Verification items for the finished model (mm, model axes). A direction names the side the tool comes from. Give positions to 0.01 mm unless a question says otherwise; leave off trailing zeros. Write each loop counter-clockwise with the first axis right and the second up, starting at its lowest first coordinate (ties: lowest second). Pieces come first, ordered by that corner, then holes.
from build123d import *

# Parameters (mm, degrees)
F0_R      = 1.2
F1_DEPTH  = 1.5
F2_DEPTH  = 5
F3_DEPTH  = 5.5
F5_DEPTH  = 2
F7_DEPTH  = 2
F8_W      = 10
F8_H      = 5
F9_DEPTH  = 1
F10_R     = 1
F11_DEPTH = 5


# Not quite as in the source:
# - a feature names something its author has since deleted; it is built from what else it names


with BuildPart() as f1:
    # F0 (on Top) → F1 (new body)
    with BuildSketch(Plane.XY):
        with BuildLine():
            Line((14.9310000289, -10.5), (14.9310000289, 10.5))
            ThreePointArc((14.9310000289, 10.5), (13.4665339264, 14.0355339264), (9.931, 15.5000000289))
            Line((9.931, 15.5000000289), (-9.931, 15.5000000289))
            ThreePointArc((-9.931, 15.5000000289), (-13.4665339264, 14.0355339264), (-14.9310000289, 10.5))
            Line((-14.9310000289, 10.5), (-14.9310000289, -10.5))
            ThreePointArc((-14.9310000289, -10.5), (-13.4665339264, -14.0355339264), (-9.931, -15.5000000289))
            Line((-9.931, -15.5000000289), (9.931, -15.5000000289))
            ThreePointArc((9.931, -15.5000000289), (13.4665339264, -14.0355339264), (14.9310000289, -10.5))
        make_face()
        with BuildLine():
            Line((-9.931, 13.5000000289), (-7.581, 13.5000000289))
            Line((-7.581, 13.5000000289), (0.069, 13.5000000289))
            Line((0.069, 13.5000000289), (4.769, 13.5000000289))
            Line((4.769, 13.5000000289), (9.931, 13.5000000289))
            ThreePointArc((9.931, 13.5000000289), (12.052320364, 12.621320364), (12.9310000289, 10.5))
            Line((12.9310000289, 10.5), (12.9310000289, -10.5))
            ThreePointArc((12.9310000289, -10.5), (12.052320364, -12.621320364), (9.931, -13.5000000289))
            Line((9.931, -13.5000000289), (4.769, -13.5000000289))
            Line((4.769, -13.5000000289), (0.069, -13.5000000289))
            Line((0.069, -13.5000000289), (-7.581, -13.5000000289))
            Line((-7.581, -13.5000000289), (-9.931, -13.5000000289))
            ThreePointArc((-9.931, -13.5000000289), (-12.052320364, -12.621320364), (-12.9310000289, -10.5))
            Line((-12.9310000289, -10.5), (-12.9310000289, -8.1))
            Line((-12.9310000289, -8.1), (-12.9310000289, 8.1))
            Line((-12.9310000289, 8.1), (-12.9310000289, 10.5))
            ThreePointArc((-12.9310000289, 10.5), (-12.052320364, 12.621320364), (-9.931, 13.5000000289))
        make_face(mode=Mode.SUBTRACT)
        with BuildLine():
            ThreePointArc((4.769, -10.45), (2.419, -8.1), (0.069, -10.45))
            ThreePointArc((0.069, -10.45), (2.419, -12.8), (4.769, -10.45))
        make_face()
        with Locations((2.419, -10.45)):
            Circle(F0_R, mode=Mode.SUBTRACT)
        with BuildLine():
            ThreePointArc((4.769, 10.45), (2.419, 12.8), (0.069, 10.45))
            ThreePointArc((0.069, 10.45), (2.419, 8.1), (4.769, 10.45))
        make_face()
        with Locations((2.419, 10.45)):
            Circle(F0_R, mode=Mode.SUBTRACT)
        with BuildLine():
            ThreePointArc((-9.931, 8.1), (-11.5927009358, 12.1117009358), (-7.581, 10.45))
            Line((-7.581, 10.45), (-7.581, 13.5000000289))
            Line((-7.581, 13.5000000289), (-9.931, 13.5000000289))
            ThreePointArc((-9.931, 13.5000000289), (-12.052320364, 12.621320364), (-12.9310000289, 10.5))
            Line((-12.9310000289, 10.5), (-12.9310000289, 8.1))
            Line((-12.9310000289, 8.1), (-9.931, 8.1))
        make_face()
        with BuildLine():
            Line((-9.931, -8.1), (-12.9310000289, -8.1))
            Line((-12.9310000289, -8.1), (-12.9310000289, -10.5))
            ThreePointArc((-12.9310000289, -10.5), (-12.052320364, -12.621320364), (-9.931, -13.5000000289))
            Line((-9.931, -13.5000000289), (-7.581, -13.5000000289))
            Line((-7.581, -13.5000000289), (-7.581, -10.45))
            ThreePointArc((-7.581, -10.45), (-11.5927009358, -12.1117009358), (-9.931, -8.1))
        make_face()
        with BuildLine():
            ThreePointArc((-7.581, -10.45), (-8.2692990642, -8.7882990642), (-9.931, -8.1))
            ThreePointArc((-9.931, -8.1), (-11.5927009358, -12.1117009358), (-7.581, -10.45))
        make_face()
        with Locations((-9.931, -10.45)):
            Circle(F0_R, mode=Mode.SUBTRACT)
        with BuildLine():
            Line((0.069, -10.45), (0.069, -13.5000000289))
            Line((0.069, -13.5000000289), (4.769, -13.5000000289))
            Line((4.769, -13.5000000289), (4.769, -10.45))
            ThreePointArc((4.769, -10.45), (2.419, -12.8), (0.069, -10.45))
        make_face()
        with BuildLine():
            ThreePointArc((-9.931, 8.1), (-8.2692990642, 8.7882990642), (-7.581, 10.45))
            ThreePointArc((-7.581, 10.45), (-11.5927009358, 12.1117009358), (-9.931, 8.1))
        make_face()
        with Locations((-9.931, 10.45)):
            Circle(F0_R, mode=Mode.SUBTRACT)
        with BuildLine():
            Line((4.769, 13.5000000289), (0.069, 13.5000000289))
            Line((0.069, 13.5000000289), (0.069, 10.45))
            ThreePointArc((0.069, 10.45), (2.419, 12.8), (4.769, 10.45))
            Line((4.769, 10.45), (4.769, 13.5000000289))
        make_face()
        with BuildLine():
            Line((-7.581, 13.5000000289), (-7.581, 10.45))
            ThreePointArc((-7.581, 10.45), (-8.2692990642, 8.7882990642), (-9.931, 8.1))
            Line((-9.931, 8.1), (-12.9310000289, 8.1))
            Line((-12.9310000289, 8.1), (-12.9310000289, -8.1))
            Line((-12.9310000289, -8.1), (-9.931, -8.1))
            ThreePointArc((-9.931, -8.1), (-8.2692990642, -8.7882990642), (-7.581, -10.45))
            Line((-7.581, -10.45), (-7.581, -13.5000000289))
            Line((-7.581, -13.5000000289), (0.069, -13.5000000289))
            Line((0.069, -13.5000000289), (0.069, -10.45))
            ThreePointArc((0.069, -10.45), (2.419, -8.1), (4.769, -10.45))
            Line((4.769, -10.45), (4.769, -13.5000000289))
            Line((4.769, -13.5000000289), (9.931, -13.5000000289))
            ThreePointArc((9.931, -13.5000000289), (12.052320364, -12.621320364), (12.9310000289, -10.5))
            Line((12.9310000289, -10.5), (12.9310000289, 10.5))
            ThreePointArc((12.9310000289, 10.5), (12.052320364, 12.621320364), (9.931, 13.5000000289))
            Line((9.931, 13.5000000289), (4.769, 13.5000000289))
            Line((4.769, 13.5000000289), (4.769, 10.45))
            ThreePointArc((4.769, 10.45), (2.419, 8.1), (0.069, 10.45))
            Line((0.069, 10.45), (0.069, 13.5000000289))
            Line((0.069, 13.5000000289), (-7.581, 13.5000000289))
        make_face()
    extrude(amount=F1_DEPTH)

    # F0 (on Top) → F2 (join)
    with BuildSketch(Plane.XY):
        with BuildLine():
            ThreePointArc((-9.931, 8.1), (-11.5927009358, 12.1117009358), (-7.581, 10.45))
            Line((-7.581, 10.45), (-7.581, 13.5000000289))
            Line((-7.581, 13.5000000289), (-9.931, 13.5000000289))
            ThreePointArc((-9.931, 13.5000000289), (-12.052320364, 12.621320364), (-12.9310000289, 10.5))
            Line((-12.9310000289, 10.5), (-12.9310000289, 8.1))
            Line((-12.9310000289, 8.1), (-9.931, 8.1))
        make_face()
        with BuildLine():
            ThreePointArc((-9.931, 8.1), (-8.2692990642, 8.7882990642), (-7.581, 10.45))
            ThreePointArc((-7.581, 10.45), (-11.5927009358, 12.1117009358), (-9.931, 8.1))
        make_face()
        with Locations((-9.931, 10.45)):
            Circle(F0_R, mode=Mode.SUBTRACT)
        with BuildLine():
            ThreePointArc((4.769, 10.45), (2.419, 12.8), (0.069, 10.45))
            ThreePointArc((0.069, 10.45), (2.419, 8.1), (4.769, 10.45))
        make_face()
        with Locations((2.419, 10.45)):
            Circle(F0_R, mode=Mode.SUBTRACT)
        with BuildLine():
            Line((4.769, 13.5000000289), (0.069, 13.5000000289))
            Line((0.069, 13.5000000289), (0.069, 10.45))
            ThreePointArc((0.069, 10.45), (2.419, 12.8), (4.769, 10.45))
            Line((4.769, 10.45), (4.769, 13.5000000289))
        make_face()
        with BuildLine():
            ThreePointArc((4.769, -10.45), (2.419, -8.1), (0.069, -10.45))
            ThreePointArc((0.069, -10.45), (2.419, -12.8), (4.769, -10.45))
        make_face()
        with Locations((2.419, -10.45)):
            Circle(F0_R, mode=Mode.SUBTRACT)
        with BuildLine():
            Line((0.069, -10.45), (0.069, -13.5000000289))
            Line((0.069, -13.5000000289), (4.769, -13.5000000289))
            Line((4.769, -13.5000000289), (4.769, -10.45))
            ThreePointArc((4.769, -10.45), (2.419, -12.8), (0.069, -10.45))
        make_face()
        with BuildLine():
            ThreePointArc((-7.581, -10.45), (-8.2692990642, -8.7882990642), (-9.931, -8.1))
            ThreePointArc((-9.931, -8.1), (-11.5927009358, -12.1117009358), (-7.581, -10.45))
        make_face()
        with Locations((-9.931, -10.45)):
            Circle(F0_R, mode=Mode.SUBTRACT)
        with BuildLine():
            Line((-9.931, -8.1), (-12.9310000289, -8.1))
            Line((-12.9310000289, -8.1), (-12.9310000289, -10.5))
            ThreePointArc((-12.9310000289, -10.5), (-12.052320364, -12.621320364), (-9.931, -13.5000000289))
            Line((-9.931, -13.5000000289), (-7.581, -13.5000000289))
            Line((-7.581, -13.5000000289), (-7.581, -10.45))
            ThreePointArc((-7.581, -10.45), (-11.5927009358, -12.1117009358), (-9.931, -8.1))
        make_face()
    extrude(amount=F2_DEPTH)

    # F0 (on Top) → F3 (join)
    with BuildSketch(Plane.XY):
        with BuildLine():
            Line((14.9310000289, -10.5), (14.9310000289, 10.5))
            ThreePointArc((14.9310000289, 10.5), (13.4665339264, 14.0355339264), (9.931, 15.5000000289))
            Line((9.931, 15.5000000289), (-9.931, 15.5000000289))
            ThreePointArc((-9.931, 15.5000000289), (-13.4665339264, 14.0355339264), (-14.9310000289, 10.5))
            Line((-14.9310000289, 10.5), (-14.9310000289, -10.5))
            ThreePointArc((-14.9310000289, -10.5), (-13.4665339264, -14.0355339264), (-9.931, -15.5000000289))
            Line((-9.931, -15.5000000289), (9.931, -15.5000000289))
            ThreePointArc((9.931, -15.5000000289), (13.4665339264, -14.0355339264), (14.9310000289, -10.5))
        make_face()
        with BuildLine():
            Line((-9.931, 13.5000000289), (-7.581, 13.5000000289))
            Line((-7.581, 13.5000000289), (0.069, 13.5000000289))
            Line((0.069, 13.5000000289), (4.769, 13.5000000289))
            Line((4.769, 13.5000000289), (9.931, 13.5000000289))
            ThreePointArc((9.931, 13.5000000289), (12.052320364, 12.621320364), (12.9310000289, 10.5))
            Line((12.9310000289, 10.5), (12.9310000289, -10.5))
            ThreePointArc((12.9310000289, -10.5), (12.052320364, -12.621320364), (9.931, -13.5000000289))
            Line((9.931, -13.5000000289), (4.769, -13.5000000289))
            Line((4.769, -13.5000000289), (0.069, -13.5000000289))
            Line((0.069, -13.5000000289), (-7.581, -13.5000000289))
            Line((-7.581, -13.5000000289), (-9.931, -13.5000000289))
            ThreePointArc((-9.931, -13.5000000289), (-12.052320364, -12.621320364), (-12.9310000289, -10.5))
            Line((-12.9310000289, -10.5), (-12.9310000289, -8.1))
            Line((-12.9310000289, -8.1), (-12.9310000289, 8.1))
            Line((-12.9310000289, 8.1), (-12.9310000289, 10.5))
            ThreePointArc((-12.9310000289, 10.5), (-12.052320364, 12.621320364), (-9.931, 13.5000000289))
        make_face(mode=Mode.SUBTRACT)
    extrude(amount=F3_DEPTH)

    # F4 (on face) → F5 (cut)
    with BuildSketch(Plane(origin=(-14.9310000289, 0, 0), x_dir=(0, -1, 0), z_dir=(-1, 0, 0))):
        with BuildLine():
            Line((7, 5.5), (-7, 5.5))
            Line((-7, 5.5), (-7, 4.75))
            ThreePointArc((-7, 4.75), (-6.8535533906, 4.3964466094), (-6.5, 4.25))
            Line((-6.5, 4.25), (6.5, 4.25))
            ThreePointArc((6.5, 4.25), (6.8535533906, 4.3964466094), (7, 4.75))
            Line((7, 4.75), (7, 5.5))
        make_face()
    extrude(amount=-F5_DEPTH, mode=Mode.SUBTRACT)

    # F6 (on face) → F7 (cut)
    with BuildSketch(Plane.YZ.offset(14.9310000289)):
        with BuildLine():
            Line((9, 2), (9, 5.5))
            Line((9, 5.5), (-9, 5.5))
            Line((-9, 5.5), (-9, 2))
            ThreePointArc((-9, 2), (-8.8535533906, 1.6464466094), (-8.5, 1.5))
            Line((-8.5, 1.5), (8.5, 1.5))
            ThreePointArc((8.5, 1.5), (8.8535533906, 1.6464466094), (9, 2))
        make_face()
    extrude(amount=-F7_DEPTH, mode=Mode.SUBTRACT)

    # F8 (on face) → F9 (join)
    with BuildSketch(Plane.XY):
        Rectangle(F8_W, F8_H)
    extrude(amount=-F9_DEPTH)

    # F10 (on face) → F11 (join)
    with BuildSketch(Plane(origin=(0, 2.5, 0), x_dir=(-1, 0, 0), z_dir=(0, 1, 0))):
        with BuildLine():
            Line((5, -1), (-5, -1))
            ThreePointArc((-5, -1), (0, -6), (5, -1))
        make_face()
        with Locations((0, -4)):
            Circle(F10_R, mode=Mode.SUBTRACT)
    extrude(amount=-F11_DEPTH)


solid = f1.part
Item 1: Scan lines: line 1 along X through (y, z) = (-4.5, 2.75); line 2 along Z through (x, y) = (-0.5, -8); line 3 along Y through (x, z) = (-4.5, 2.75). Record each from-to range of solid material in increasing order.
Answer key:
line 1: x = -14.93 to -12.93
line 2: z = 0 to 1.5
line 3: y = -15.5 to -13.5, 13.5 to 15.5
Item 2: Release check for a two-part mould opening along Y. For faces 1 (the face through (13.5, 14, 2.7)), 2 (the face through (2.5, -8.1, 3.2)), 3 (the face through (5, 0, -0.5)) record: released by +Y, released by -Y, zero draft, split by the parting line, or undercut.
Answer key:
face 1: released by +Y
face 2: undercut
face 3: zero draft
Item 3: Set-up check for faces 4 (the face through (-10.19, 9.28, 2.46)), 5 (the face through (14, 9, 4)), 6 (the face through (-14, 0, 4.25)), 7 (the face through (0.069, 12, 3)): record each of +Z, -Z, +X, -X, +Y, -Y from which the full face is reachable in a straight line by a thin tool's end or side.
Answer key:
face 4: +Z, -Z
face 5: +Z, +X
face 6: +Z, +X, -X
face 7: +Z
Item 4: Sectioned sample at A-A on z = -4. Record the cut outline in (x, y), then the cut area to 3 significant figures.
Answer key:
outline: (-4, -2.5) - (-1, -2.5) - (-1, 2.5) - (-4, 2.5) - close; (1, -2.5) - (4, -2.5) - (4, 2.5) - (1, 2.5) - close
area: 30.0 mm2
Item 5: Depth check by flat-ended pin: pin 1 (6 mm diameter, centred on x = -9.5, y = 11.5, fed in from +Z); pin 2 (1.5 mm diameter, centred on x = -8, y = 7, fed in from +Z); pin 3 (3 mm diameter, centred on x = -9.931, y = -10.45, fed in from -Z); pin 4 (3 mm diameter, centred on x = -9.931, y = 10.45, fed in from +Z). Enter the tip coordinate at first touch or a pass-through.
Answer key:
pin 1: stops at z = 5.5
pin 2: stops at z = 1.5
pin 3: stops at z = 0
pin 4: stops at z = 5
Item 6: Sectioned sample at D-D on y = 5. Record the cut outline in (x, z), then the cut area to 3 significant figures.
Answer key:
outline: (-14.93, 0) - (14.93, 0) - (14.93, 1.5) - (-12.93, 1.5) - (-12.93, 4.25) - (-14.93, 4.25) - close
area: 50.3 mm2
Item 7: Sectioned sample at B-B on y = -1. Record the cut outline in (x, z), then the cut area to 3 significant figures.
Answer key:
outline: (-14.93, 0) - (-5, 0) - (-5, -1) arc R5 ccw to (5, -1) - (5, 0) - (14.93, 0) - (14.93, 1.5) - (-12.93, 1.5) - (-12.93, 4.25) - (-14.93, 4.25) - close; hole circle Ø2 at (0, -4)
area: 96.4 mm2
Item 8: Sectioned sample at C-C on x = -0.5. Record the cut outline in (y, z), then the cut area to 3 significant figures.
Answer key:
outline: (-15.5, 0) - (-2.5, 0) - (-2.5, -3.13) - (2.5, -3.13) - (2.5, 0) - (15.5, 0) - (15.5, 5.5) - (13.5, 5.5) - (13.5, 1.5) - (-13.5, 1.5) - (-13.5, 5.5) - (-15.5, 5.5) - close; (-2.5, -5.97) - (2.5, -5.97) - (2.5, -4.87) - (-2.5, -4.87) - close
area: 83.7 mm2
